```python
from build123d import *

# Parameters (mm, degrees)
SKETCH1_W           = 40
SKETCH1_H           = 30
BOSS_EXTRUDE1_DEPTH = 4
SKETCH3_R           = 2.55
CUT_EXTRUDE2_DEPTH  = 26.317977802
CHAMFER1_SIZE       = 3
LPATTERN1_COUNT     = 2
LPATTERN1_PITCH     = 20


with BuildPart() as part:
    # Sketch1 → Boss-Extrude1 (new body)
    with BuildSketch(Plane.XY):
        Rectangle(SKETCH1_W, SKETCH1_H)
    extrude(amount=BOSS_EXTRUDE1_DEPTH)

    # Sketch3 → Cut-Extrude2 (cut, through all)
    with BuildSketch(Plane.XY.offset(4)):
        with Locations((10, 7.5)):
            Circle(SKETCH3_R)
        with Locations((10, -7.5)):
            Circle(SKETCH3_R)
    cut_extrude2 = extrude(amount=-CUT_EXTRUDE2_DEPTH, mode=Mode.SUBTRACT)

    # Chamfer1
    chamfer1_edges = [part.edges().sort_by_distance(p)[0] for p in [
        (20, -15, 2),
        (-20, -15, 2),
        (-20, 15, 2),
        (20, 15, 2),
    ]]
    chamfer(chamfer1_edges, length=CHAMFER1_SIZE)

    # LPattern1: Cut-Extrude2 ×2
    with Locations(*[(-i * LPATTERN1_PITCH, 0, 0) for i in range(1, LPATTERN1_COUNT)]):
        add(cut_extrude2, mode=Mode.SUBTRACT)


solid = part.part
```
Read the model definition and answer for the solid it produces. Units are mm, in the model's axes. Coordinates: 2 decimals unless noted, no trailing zeros. Write each loop counter-clockwise with the first axis right and the second up, starting at its lowest first coordinate (ties: lowest second). Pieces come first, ordered by that corner, then holes. Notation, with made-up numbers: (10, 28.25) -> (35, 28.25) arc R9 cw to (35, 34.25) -> close; hole circle Ø6 at (35.5, -35). An arc over 180 degrees is marked (long way). Write item = value, one per line.
(1) Straight lines are drawn through the part: L1, parallel to Y at x = 10, z = 3.55; L2, parallel to Y at x = 8.5, z = 1.8; L3, parallel to X at y = 8.25, z = 2.25. For each, find the intervals that lie inside material, in ascending order. Write a range as from..to.
From the geometry:
L1 = -15..-10.05, -4.95..4.95, 10.05..15
L2 = -15..-9.56, -5.44..5.44, 9.56..15
L3 = -20..-12.44, -7.56..7.56, 12.44..20
(2) Section B-B on y = -7.5 is taken. Write down the section's boundary in (x, z).
From the geometry:
outline = (-20, 0) -> (-12.55, 0) -> (-12.55, 4) -> (-20, 4) -> close; (-7.45, 0) -> (7.45, 0) -> (7.45, 4) -> (-7.45, 4) -> close; (12.55, 0) -> (20, 0) -> (20, 4) -> (12.55, 4) -> close
(3) For a pull along X with two mould halves and no side action, classify faces 1 (the face through (20, 0, 2)), 2 (the face through (-18, -14, 2)), 3 (the face through (11.18, -9.76, 2.03)) as +X half, -X half, draft (parallel to the pull), parting line (faces both ways), or undercut.
From the geometry:
face_1 = +X half
face_2 = -X half
face_3 = undercut
(4) Given pin 1 Ø1 at (x, y) = (-4, -7.5) entering from -Z, flat-ended and moving along its own axis, determine where the tip first touches the part or whether it passes through.
From the geometry:
pin_1 = 0
(5) Section A-A on x = -10 is taken. Write down the section's boundary in (y, z).
From the geometry:
outline = (-15, 0) -> (-10.05, 0) -> (-10.05, 4) -> (-15, 4) -> close; (-4.95, 0) -> (4.95, 0) -> (4.95, 4) -> (-4.95, 4) -> close; (10.05, 0) -> (15, 0) -> (15, 4) -> (10.05, 4) -> close
(6) Section C-C on z = 3.3 is taken. Write down the section's boundary in (x, y).
From the geometry:
outline = (-20, -12) -> (-17, -15) -> (17, -15) -> (20, -12) -> (20, 12) -> (17, 15) -> (-17, 15) -> (-20, 12) -> close; hole circle Ø5.1 at (-10, -7.5); hole circle Ø5.1 at (-10, 7.5); hole circle Ø5.1 at (10, -7.5); hole circle Ø5.1 at (10, 7.5)
